Verification items for the finished model (mm, model axes). Give positions to 0.01 mm unless a question says otherwise; leave off trailing zeros. Loops run counter-clockwise (first coordinate to the right, second up) from the corner with the lowest first, then second, coordinate; pieces in that order, holes last. Notation, with made-up numbers: M 76.25,9 L 82.25,9 A22 ccw 82.25,45 Z; hole C -10.5,22 d3. An arc over 180 degrees is marked long. Put each result on its own line as item: value. Start each with the question number.
from build123d import *

# Parameters (mm, degrees)
F1_DEPTH = 3.048


with BuildPart() as f1:
    # F0 (on Front) → F1 (new body)
    with BuildSketch(Plane.XZ):
        Polygon((-6.500012, -74.500003), (-6.500012, -71.500009), (3.499993, -71.500009), (3.499993, -74.500003), (14.999995, -74.500003), (14.999995, -54.999992), (12.000001, -54.999992), (12.000001, -45.000012), (14.999995, -45.000012), (14.999995, -4.99999), (12.000001, -4.99999), (12.000001, 4.99999), (14.999995, 4.99999), (14.999995, 45.000012), (12.000001, 45.000012), (12.000001, 54.999992), (14.999995, 54.999992), (14.999995, 74.500003), (3.499993, 74.500003), (3.499993, 71.500009), (-6.500012, 71.500009), (-6.500012, 74.500003), (-14.999995, 74.500003), (-14.999995, -74.500003), align=None)
    extrude(amount=F1_DEPTH)


solid = f1.part
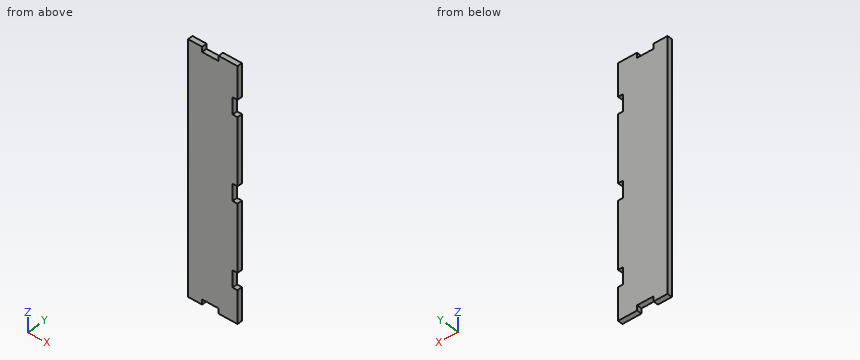
Q1. Go/stop test with flat-tipped pins: pin 1 (0.9 mm diameter, centred on y = -2, z = 0, fed in from +X); pin 2 (1.5 mm diameter, centred on x = -5.5, y = -0.5, fed in from -Z); pin 3 (1 mm diameter, centred on x = -5.5, y = -1.5, fed in from +Z). Record where each tip stops, or that it passes through.
Q2. Scan lines: L1, parallel to Z at x = 0.25, y = -1.6; L2, parallel to X at y = -0.75, z = -3. Record each from-to range of solid material in increasing order.
Q3. Cross-section at C-C, the plane x = -0.25. Record the boundary of the cut face in (y, z), then the cut area to 3 significant figures.
Q4. Cross-section at B-B, the plane z = -47.5. Record the boundary of the cut face in (x, y).
Q5. Cross-section at A-A, the plane y = -1.8. Record the boundary of the cut face in (x, z), then the cut area to 3 significant figures.
Ans:
1. pin 1: stops at x = 12
1. pin 2: stops at z = -71.5
1. pin 3: stops at z = 71.5
2. L1: z = -71.5 to 71.5
2. L2: x = -15 to 12
3. outline: M -3.05,-71.5 L 0,-71.5 L 0,71.5 L -3.05,71.5 Z
3. area: 436 mm^2
4. outline: M -15,-3.05 L 12,-3.05 L 12,0 L -15,0 Z
5. outline: M -15,-74.5 L -6.5,-74.5 L -6.5,-71.5 L 3.5,-71.5 L 3.5,-74.5 L 15,-74.5 L 15,-55 L 12,-55 L 12,-45 L 15,-45 L 15,-5 L 12,-5 L 12,5 L 15,5 L 15,45 L 12,45 L 12,55 L 15,55 L 15,74.5 L 3.5,74.5 L 3.5,71.5 L -6.5,71.5 L -6.5,74.5 L -15,74.5 Z
5. area: 4,320 mm^2
